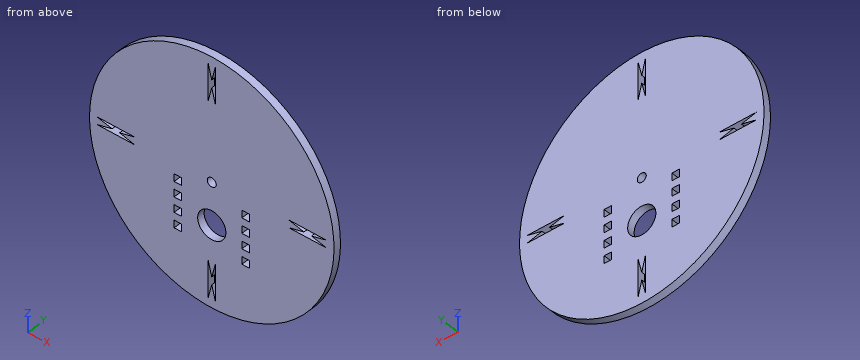
from build123d import *

# Parameters (mm, degrees)
SKETCH1_R           = 82.55
SKETCH1_R_2         = 3.048
SKETCH1_R_3         = 9.525
SKETCH1_W           = 5.08
SKETCH1_H           = 5.08
BOSS_EXTRUDE1_DEPTH = 5.08
CUT_EXTRUDE1_DEPTH  = 5.08


with BuildPart() as part:
    # Sketch1 → Boss-Extrude1 (new body)
    with BuildSketch(Plane(origin=(0, 0, 0), x_dir=(1, 0, 0), z_dir=(0, 1, 0))):
        with Locations(Location((-62.967414891, 81.40064069, 0), (0, 0, 270))):
            Circle(SKETCH1_R)
        with Locations(Location((-62.967414891, 81.40064069, 0), (0, 0, 270))):
            Circle(SKETCH1_R_2, mode=Mode.SUBTRACT)
        with Locations(Location((-62.967414891, 109.55654069, 0), (0, 0, 270))):
            Circle(SKETCH1_R_3, mode=Mode.SUBTRACT)
        with Locations((-85.827414891, 111.88064069)):
            Rectangle(SKETCH1_W, SKETCH1_H, mode=Mode.SUBTRACT)
        with Locations((-85.827414891, 91.56064069)):
            Rectangle(SKETCH1_W, SKETCH1_H, mode=Mode.SUBTRACT)
        with Locations((-85.827414891, 101.72064069)):
            Rectangle(SKETCH1_W, SKETCH1_H, mode=Mode.SUBTRACT)
        with Locations((-85.827414891, 122.04064069)):
            Rectangle(SKETCH1_W, SKETCH1_H, mode=Mode.SUBTRACT)
        with Locations((-40.107414891, 122.04064069)):
            Rectangle(SKETCH1_W, SKETCH1_H, mode=Mode.SUBTRACT)
        with Locations((-40.107414891, 111.88064069)):
            Rectangle(SKETCH1_W, SKETCH1_H, mode=Mode.SUBTRACT)
        with Locations((-40.107414891, 101.72064069)):
            Rectangle(SKETCH1_W, SKETCH1_H, mode=Mode.SUBTRACT)
        with Locations((-40.107414891, 91.56064069)):
            Rectangle(SKETCH1_W, SKETCH1_H, mode=Mode.SUBTRACT)
    extrude(amount=BOSS_EXTRUDE1_DEPTH)

    # Sketch2 → Cut-Extrude1 (cut)
    with BuildSketch(Plane(origin=(0, 5.08, 0), x_dir=(1, 0, 0), z_dir=(0, 1, 0))):
        Polygon((-62.967414891, 148.71064069), (-60.427414891, 158.87064069), (-60.427414891, 133.47064069), (-62.967414891, 143.63064069), (-65.507414891, 133.47064069), (-65.507414891, 158.87064069), align=None)
        Polygon((4.342585109, 81.40064069), (14.502585109, 78.86064069), (-10.897414891, 78.86064069), (-0.737414891, 81.40064069), (-10.897414891, 83.94064069), (14.502585109, 83.94064069), align=None)
        Polygon((-62.967414891, 14.09064069), (-65.507414891, 3.93064069), (-65.507414891, 29.33064069), (-62.967414891, 19.17064069), (-60.427414891, 29.33064069), (-60.427414891, 3.93064069), align=None)
        Polygon((-130.277414891, 81.40064069), (-140.437414891, 83.94064069), (-115.037414891, 83.94064069), (-125.197414891, 81.40064069), (-115.037414891, 78.86064069), (-140.437414891, 78.86064069), align=None)
    extrude(amount=-CUT_EXTRUDE1_DEPTH, mode=Mode.SUBTRACT)


solid = part.part
Design review of the part built by this model. Coordinates are the model's own, in mm. Round coordinates to 2 decimals unless told otherwise and drop trailing zeros. Write each loop counter-clockwise with the first axis right and the second up, starting at its lowest first coordinate (ties: lowest second). Pieces come first, ordered by that corner, then holes. Notation, with made-up numbers: (17.5, -20.75) -> (30.5, -20.75) arc R26 cw to (30.5, -0.75) -> close; hole circle Ø3 at (30.5, 79.25). An arc over 180 degrees is marked (long way). One line per item, written item: value. Start each with the question number.
Q1. Add section B-B (x = -56.5). Give the boundary of the cut face in (y, z), then the cut area to 3 significant figures.
Q2. Add section A-A (x = 7). Give the boundary of the cut face in (y, z) (3 decimals).
Q3. To check wall thickness, follow probe 1 along Z at (x, y) = (-116, 0.25); probe 2 along X at (y, z) = (4.65, -6); probe 3 along X at (y, z) = (3.3, -122). State the ranges of each line that lie inside material, in increasing order.
Q4. Add section C-C (y = 1.5). State how many separate pieces and enclosed holes the cut face has, then the cut area to 3 significant figures.
Q5. Add section D-D (z = -36.5). Give the boundary of the cut face in (x, y), then the cut area to 3 significant figures.
Q6. Insertion check: P1, Ø2.5, axis at y = 3, z = -122.5, coming from the -X side; P2, Ø1.5, axis at y = 4, z = -112.5, coming from the +X side; P3, Ø1.5, axis at x = -86, y = 3, coming from the -Z side; P4, Ø10, axis at x = -97, z = -57.5, coming from the -Y side. Each pin has a flat end and moves straight along its axis. Give the tip position at first contact, or say it passes through.
Response:
1. outline: (0, -163.7) -> (5.08, -163.7) -> (5.08, -116.55) -> (0, -116.55) -> close; (0, -102.56) -> (5.08, -102.56) -> (5.08, 0.9) -> (0, 0.9) -> close
1. area: 765 mm^2
2. outline: (0, -125.208) -> (5.08, -125.208) -> (5.08, -83.941) -> (0, -83.941) -> close; (0, -82.065) -> (5.08, -82.065) -> (5.08, -80.736) -> (0, -80.736) -> close; (0, -78.861) -> (5.08, -78.861) -> (5.08, -37.594) -> (0, -37.594) -> close
3. probe 1: z = -144.66 to -83.94, -83.7 to -79.1, -78.86 to -18.14
3. probe 2: x = -96.57 to -65.51, -64.99 to -60.94, -60.43 to -29.36
3. probe 3: x = -134.84 to -88.37, -83.29 to -42.65, -37.57 to 8.91
4. separate pieces: 1
4. enclosed holes: 14
4. area: 20,600 mm^2
5. outline: (-132.24, 0) -> (6.3, 0) -> (6.3, 5.08) -> (-132.24, 5.08) -> close
5. area: 704 mm^2
6. P1: stops at x = -135.26
6. P2: stops at x = 13.8
6. P3: stops at z = -160.89
6. P4: stops at y = 0
